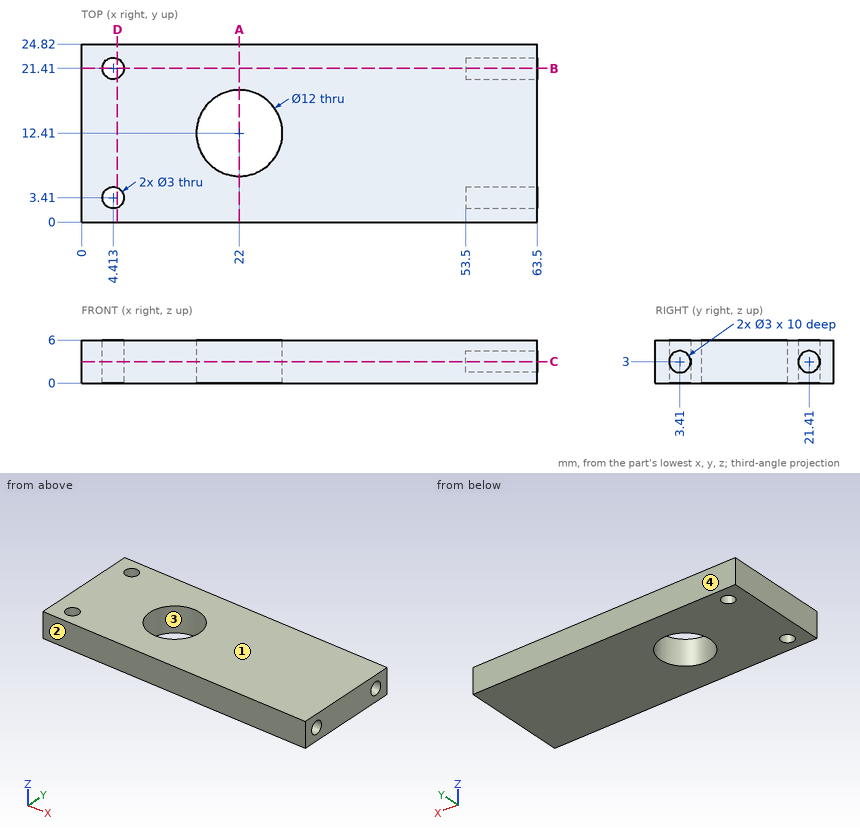
Can you work these out from the drawing? Everything is in mm from the part's minimum corner. Round coordinates to 2 decimals unless told otherwise and drop trailing zeros. Loops run counter-clockwise (first coordinate to the right, second up) from the corner with the lowest first, then second, coordinate; pieces in that order, holes last. Notation, with made-up numbers: (-7, 14) - (43, 14) arc R22 ccw to (43, 24) - close; hole circle Ø8 at (56.25, -7.5). An arc over 180 degrees is marked (long way). Write item = value, one per line. Start each with the question number.
(1) If we section it at D-D (x = 5): Please give me the cut outline in (y, z), and give its area (3 significant figures).
(2) For P1, Ø0.9, axis at y = 3, z = 3.5, coming from the +X side, with a flat end and sliding along its axis, tell me the tip position at first contact or that it passes through.
(3) If I drill on probe 1 along Y at (x, z) = (58.75, 3); probe 2 along Y at (x, z) = (22, 2.2); probe 3 along Z at (x, y) = (58, 4.5), over which ranges is the centre line in solid material (lowest first)? Write a range as [from, to].
(4) If we section it at A-A (x = 22): Please give me the cut outline in (y, z).
(5) If we mould it in two halves opening along Y, with no side actions, what happens to the marked faces 1, 2, 3 and 4? For each: released by +Y, released by -Y, zero draft, split by the parting line, or undercut.
(6) If we section it at B-B (y = 21.41): Please give me the cut outline in (x, z).
(7) If we section it at C-C (z = 3): Please give me the cut outline in (x, y).
Ans:
q1.outline = (0, 0) - (2.03, 0) - (2.03, 6) - (0, 6) - close; (4.79, 0) - (20.03, 0) - (20.03, 6) - (4.79, 6) - close; (22.79, 0) - (24.82, 0) - (24.82, 6) - (22.79, 6) - close
q1.area = 116 mm²
q2.P1 = 53.5
q3.probe_1 = [0, 1.91], [4.91, 19.91], [22.91, 24.82]
q3.probe_2 = [0, 6.41], [18.41, 24.82]
q3.probe_3 = [0, 1.97], [4.03, 6]
q4.outline = (0, 0) - (6.41, 0) - (6.41, 6) - (0, 6) - close; (18.41, 0) - (24.82, 0) - (24.82, 6) - (18.41, 6) - close
q5.face_1 = zero draft
q5.face_2 = released by -Y
q5.face_3 = undercut
q5.face_4 = released by +Y
q6.outline = (0, 0) - (2.91, 0) - (2.91, 6) - (0, 6) - close; (5.91, 0) - (63.5, 0) - (63.5, 1.5) - (53.5, 1.5) - (53.5, 4.5) - (63.5, 4.5) - (63.5, 6) - (5.91, 6) - close
q7.outline = (0, 0) - (63.5, 0) - (63.5, 1.91) - (53.5, 1.91) - (53.5, 4.91) - (63.5, 4.91) - (63.5, 19.91) - (53.5, 19.91) - (53.5, 22.91) - (63.5, 22.91) - (63.5, 24.82) - (0, 24.82) - close; hole circle Ø3 at (4.41, 3.41); hole circle Ø3 at (4.41, 21.41); hole circle Ø12 at (22, 12.41)
